Geometry: final body of the model. Coordinates: model frame, mm. A direction names the side the tool comes from. Give positions to 0.01 mm unless a question says otherwise; leave off trailing zeros. Order: outer loops, then holes, each group sorted by start corner. A loop starts at its lowest first (then second) coordinate and runs counter-clockwise, first axis right, second up. Notation, with made-up numbers: (-26, 21) - (-16, 21) arc R35 ccw to (-16, 56) - close; hole circle Ø7 at (-16.75, 27). An arc over 180 degrees is marked (long way). Put each result on its own line as item: value. Start each with the question number.
1. Section D-D on y = 45. Return the cut outline in (x, z), plus the area to 3 significant figures.
2. Set-up query: faces 1 (the flat face through (-10.739, -37.494, 1.873)), 2 (the flat face through (-38.977, -1.373, 1.873)), 3 (the flat face through (36.11, -13.64, 1.87)). Return all of +Z, -Z, +X, -X, +Y, -Y with unobstructed straight access to the full face (end or side cutting, diameter ignored); none if empty.
3. Section B-B on y = -48.5. Return the cut outline in (x, z).
4. Section A-A on x = -47.5. Return the cut outline in (y, z), plus the area to 3 significant figures.
5. Section C-C on z = 0.7. Return the cut outline in (x, y).
6. First-contact query: P1, Ø1.5, axis at y = 12.5, z = 1, coming from the +X side. Flat tip, straight axial feed; report the tip coordinate or a pass-through.
7. Ray query, line 1 along Y through (x, z) = (25, 0.45); line 2 along Y through (x, z) = (23, 3.5); line 3 along X through (y, z) = (26, 0.9). Return the intervals inside material, ascending. Write a range as from..to.
8. Mould query, pull axis X, two halves, no side actions, for faces 4 (the flat face through (24.13, 30.13, 1.87)), 5 (the flat face through (2, 4, 3.8)), 6 (the flat face through (-44.36, 36.29, 1.87)). Classes: pulls with the +X half, pulls with the -X half, needs draft (parallel to the pull), parting line crosses it, or undercut.
Autodesk Fusion 360 part; units mm, degrees
sketch "Sketch1" plane through (0, 0, 0) normal (0, 0, 1) x (1, 0, 0)
  line L0 (17.5654, 17.3955) -> (-11.1161, 22.0812)
  line L1 (-11.1161, 22.0812) -> (-24.4355, -3.7486)
  line L2 (-24.4355, -3.7486) -> (-3.9858, -24.3979)
  line L3 (-3.9858, -24.3979) -> (21.9721, -11.3301)
  line L4 (21.9721, -11.3301) -> (17.5654, 17.3955)
  line L5 (17.5654, 17.3955) -> (21.9721, -11.3301)
  line L6 (21.9721, -11.3301) -> (50.6536, -16.0158)
  line L7 (50.6536, -16.0158) -> (63.973, 9.814)
  line L8 (63.973, 9.814) -> (43.5233, 30.4633)
  line L9 (43.5233, 30.4633) -> (17.5654, 17.3955)
  line L10 (17.5654, 17.3955) -> (30.8847, 43.2253)
  line L11 (30.8847, 43.2253) -> (10.4351, 63.8746)
  line L12 (10.4351, 63.8746) -> (-15.5229, 50.8068)
  line L13 (-15.5229, 50.8068) -> (-11.1161, 22.0812)
  line L14 (-11.1161, 22.0812) -> (17.5654, 17.3955)
  line L15 (-11.1161, 22.0812) -> (-31.5658, 42.7305)
  line L16 (-31.5658, 42.7305) -> (-57.5237, 29.6627)
  line L17 (-57.5237, 29.6627) -> (-53.117, 0.937)
  line L18 (-53.117, 0.937) -> (-24.4355, -3.7486)
  line L19 (-24.4355, -3.7486) -> (-11.1161, 22.0812)
  line L20 (-24.4355, -3.7486) -> (-50.3935, -16.8164)
  line L21 (-50.3935, -16.8164) -> (-45.9867, -45.542)
  line L22 (-45.9867, -45.542) -> (-17.3052, -50.2277)
  line L23 (-17.3052, -50.2277) -> (-3.9858, -24.3979)
  line L24 (-3.9858, -24.3979) -> (-24.4355, -3.7486)
  line L25 (-3.9858, -24.3979) -> (0.4209, -53.1236)
  line L26 (0.4209, -53.1236) -> (29.1024, -57.8092)
  line L27 (29.1024, -57.8092) -> (42.4218, -31.9795)
  line L28 (42.4218, -31.9795) -> (21.9721, -11.3301)
  line L29 (21.9721, -11.3301) -> (-3.9858, -24.3979)
  point P0 (39.5375, 6.0654)
  point P1 (6.4492, 39.4767)
  point P2 (-35.5516, 18.3326)
  point P3 (-28.4213, -28.1465)
  point P4 (17.9863, -35.7281)
  dimension "d1" = 20
extrude "Extrude1" add sketch "Sketch1" along normal blind 3.8
sketch "Sketch2" plane through (0, 0, 3.8) normal (0, 0, 1) x (-1, 0, 0)
  line L0 (-42.4218, 31.9795) -> (-21.9721, 11.3301)
  line L1 (-21.9721, 11.3301) -> (-50.6536, 16.0158)
  line L2 (-50.6536, 16.0158) -> (-63.973, -9.814)
  line L3 (-63.973, -9.814) -> (-43.5233, -30.4633)
  line L4 (-43.5233, -30.4633) -> (-17.5654, -17.3955)
  line L5 (-17.5654, -17.3955) -> (-30.8847, -43.2253)
  line L6 (-30.8847, -43.2253) -> (-10.4351, -63.8746)
  line L7 (-10.4351, -63.8746) -> (15.5229, -50.8068)
  line L8 (15.5229, -50.8068) -> (11.1161, -22.0812)
  line L9 (11.1161, -22.0812) -> (31.5658, -42.7305)
  line L10 (31.5658, -42.7305) -> (57.5237, -29.6627)
  line L11 (57.5237, -29.6627) -> (53.117, -0.937)
  line L12 (53.117, -0.937) -> (24.4355, 3.7486)
  line L13 (24.4355, 3.7486) -> (50.3935, 16.8164)
  line L14 (50.3935, 16.8164) -> (45.9867, 45.542)
  line L15 (45.9867, 45.542) -> (17.3052, 50.2277)
  line L16 (17.3052, 50.2277) -> (3.9858, 24.3979)
  line L17 (3.9858, 24.3979) -> (-0.4209, 53.1236)
  line L18 (-0.4209, 53.1236) -> (-29.1024, 57.8092)
  line L19 (-29.1024, 57.8092) -> (-42.4218, 31.9795)
Resolved:
1. outline: (-14.63, 0) - (29.13, 0) - (29.13, 3.8) - (-14.63, 3.8) - close
1. area: 166 mm^2
2. face 1: +Z, -Z, -Y
2. face 2: +Z, -Z, -X
2. face 3: +Z, -Z
3. outline: (-27.88, 0) - (-16.41, 0) - (-16.41, 3.8) - (-27.88, 3.8) - close; (-0.29, 0) - (33.9, 0) - (33.9, 3.8) - (-0.29, 3.8) - close
4. outline: (-35.68, 0) - (-15.36, 0) - (-15.36, 3.8) - (-35.68, 3.8) - close; (0.02, 0) - (34.71, 0) - (34.71, 3.8) - (0.02, 3.8) - close
4. area: 209 mm^2
5. outline: (-57.52, 29.66) - (-53.12, 0.94) - (-24.44, -3.75) - (-50.39, -16.82) - (-45.99, -45.54) - (-17.31, -50.23) - (-3.99, -24.4) - (0.42, -53.12) - (29.1, -57.81) - (42.42, -31.98) - (21.97, -11.33) - (50.65, -16.02) - (63.97, 9.81) - (43.52, 30.46) - (17.57, 17.4) - (30.88, 43.23) - (10.44, 63.87) - (-15.52, 50.81) - (-11.12, 22.08) - (-31.57, 42.73) - close
6. P1: x = 62.06
7. line 1: -57.14..-14.39, -11.82..21.14, 31.81..49.17
7. line 2: -56.81..-12.37, -11.5..20.13, 27.93..51.19
7. line 3: -56.96..-15, -11.72..22, 34.66..47.94
8. face 4: undercut
8. face 5: needs draft
8. face 6: pulls with the -X half
